Can you work these out from the model? Positions are in its coordinate system, mm. Face numbers are marked on the shaded views. A direction names the side the tool comes from. Round coordinates to 2 decimals unless told otherwise and drop trailing zeros. Order: outer loops, then holes, each group sorted by start corner. A loop starts at its lowest first (then second) coordinate and runs counter-clockwise, first axis right, second up. Notation, with made-up numbers: M 18.5,-35 L 23.5,-35 A29 cw 23.5,-6 Z; hole C 76,75.25 d5. An arc over 180 degrees is marked long. Answer as CSV lines item,"result". Start each with the question number.
from build123d import *

# Parameters (mm, degrees)
SKETCH1_R           = 7
SKETCH1_R_2         = 4.075
BOSS_EXTRUDE1_DEPTH = 7
SKETCH2_R           = 5.95
BOSS_EXTRUDE2_DEPTH = 1.5
SKETCH3_R           = 5.95
SKETCH3_W           = 10.3
SKETCH3_H           = 10.3
BOSS_EXTRUDE3_DEPTH = 5
SKETCH4_R           = 1.4
CUT_EXTRUDE2_DEPTH  = 10


with BuildPart() as part:
    # Sketch1 → Boss-Extrude1 (new body)
    with BuildSketch(Plane.XY):
        with Locations((-3.892264878, 1.820575507)):
            Circle(SKETCH1_R)
        with Locations((-3.892264878, 1.820575507)):
            Circle(SKETCH1_R_2, mode=Mode.SUBTRACT)
    extrude(amount=BOSS_EXTRUDE1_DEPTH)

    # Sketch2 → Boss-Extrude2 (add)
    with BuildSketch(Plane.XY.offset(7)):
        with Locations((-3.892264878, 1.820575507)):
            Circle(SKETCH2_R)
    extrude(amount=BOSS_EXTRUDE2_DEPTH)

    # Sketch3 → Boss-Extrude3 (add)
    with BuildSketch(Plane.XY.offset(8.5)):
        with Locations((-3.892264878, 1.820575507)):
            Circle(SKETCH3_R)
        with Locations((4.316754573, 1.820575507)):
            Rectangle(SKETCH3_W, SKETCH3_H)
    extrude(amount=BOSS_EXTRUDE3_DEPTH)

    # Sketch4 → Cut-Extrude2 (cut)
    with BuildSketch(Plane(origin=(9.466754573, 0, 0), x_dir=(0, 0, -1), z_dir=(1, 0, 0))):
        with Locations((-3.5, 1.870575507)):
            Circle(SKETCH4_R)
    extrude(amount=-CUT_EXTRUDE2_DEPTH, mode=Mode.SUBTRACT)


solid = part.part
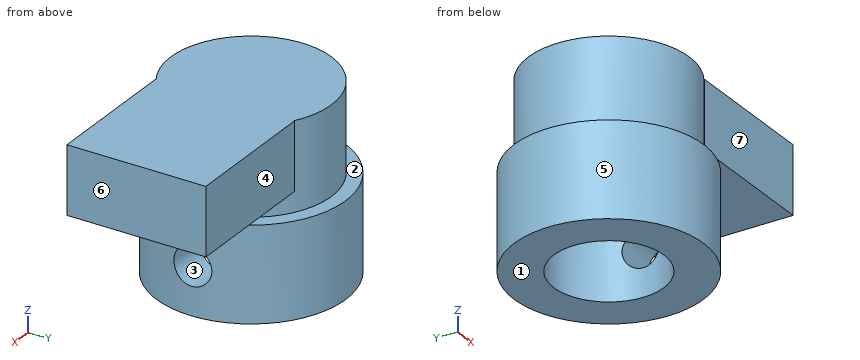
(1) I want a section at A-A on y = 3. Write out the boundary of the cut face in (x, z), and give its area (3 significant figures).
(2) I want a section at D-D on y = -1.5. Write out the boundary of the cut face in (x, z).
(3) If I drill on line 1 along Z through (x, y) = (2.25, 4.5); line 2 along Y through (x, z) = (-4, 1); line 3 along Y through (x, z) = (1.8, 3.5), over which ranges is the centre line in solid material (lowest first)?
(4) I want a section at C-C on x = 6. Write out the boundary of the cut face in (y, z), and give its area (3 significant figures).
(5) I want a section at B-B on z = 10.25. Write out the boundary of the cut face in (x, y), and give its area (3 significant figures).
(6) If we mould it in two halves opening along Z, with no side actions, what happens to the marked faces 1, 2, 3 and 4? For each: +Z half, -Z half, draft (parallel to the pull), parting line (faces both ways), or undercut.
(7) For the marked faces 5, 6 and 7, which set-ups out of +Z, -Z, +X, -X, +Y, -Y let a thin tool reach every point of the face, with its end or its side?
(8) I'm going to push flat-ended pins straight in: P1, Ø1.5, axis at x = -4, z = 9.5, coming from the -Y side; P2, Ø1.5, axis at x = 6.5, z = 12, coming from the -Y side; P3, Ø2.5, axis at x = 4, z = 10, coming from the +Y side. Where does each tip first touch, or does it pass through?
From the geometry:
1,outline,"M -10.79,0 L -7.79,0 L -7.79,7 L 0.01,7 L 0.01,4.33 L 3.01,4.33 L 3.01,7 L 1.94,7 L 1.94,8.5 L 9.47,8.5 L 9.47,13.5 L -9.72,13.5 L -9.72,7 L -10.79,7 Z; M 0.01,0 L 3.01,0 L 3.01,2.67 L 0.01,2.67 Z"
1,area,"150 mm²"
2,outline,"M -10.05,0 L -6.25,0 L -6.25,7 L -1.53,7 L -1.53,0 L 2.27,0 L 2.27,7 L 1.04,7 L 1.04,8.5 L 9.47,8.5 L 9.47,13.5 L -8.83,13.5 L -8.83,7 L -10.05,7 Z"
3,line 1,"0 to 7, 8.5 to 13.5"
3,line 2,"-5.18 to -2.25, 5.89 to 8.82"
3,line 3,"-2.25 to 0.47, 3.27 to 5.89"
4,outline,"M -3.33,8.5 L 6.97,8.5 L 6.97,13.5 L -3.33,13.5 Z"
4,area,"51.5 mm²"
5,outline,"M -0.83,-3.33 L 9.47,-3.33 L 9.47,6.97 L -0.83,6.97 L -0.83,6.92 A5.95 ccw long -0.83,-3.28 Z"
5,area,"196 mm²"
6,face 1,"-Z half"
6,face 2,"undercut"
6,face 3,"undercut"
6,face 4,"draft"
7,face 5,"-Z"
7,face 6,"+Z, -Z, +X, +Y, -Y"
7,face 7,"+Z, +X, -Y"
8,P1,"y = -4.13"
8,P2,"y = -3.33"
8,P3,"y = 6.97"
